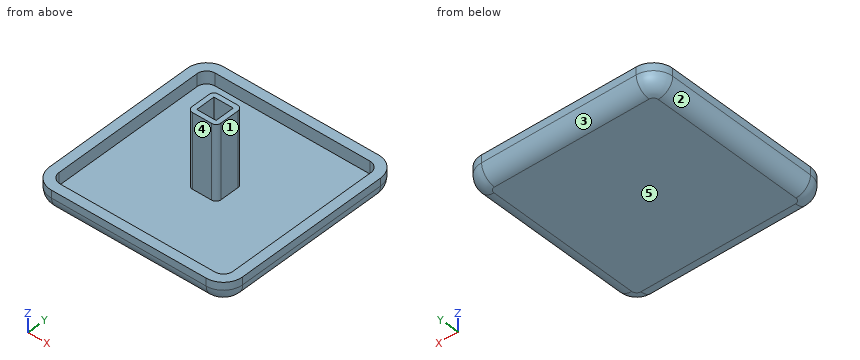
Autodesk Inventor part; units mm, degrees
ref_plane "YZ Plane" through (0, 0, 0) normal (1, 0, 0) x (0, 1, 0)
ref_plane "XZ Plane" through (0, 0, 0) normal (0, 1, 0) x (-1, 0, 0)
ref_plane "XY Plane" through (0, 0, 0) normal (0, 0, 1) x (1, 0, 0)
sketch "Skizze1" plane through (0, 0, 0) normal (0, 0, 1) x (1, 0, 0)
  line L0 (-10, 10) -> (10, 10)
  line L1 (10, 10) -> (10, -10)
  line L2 (10, -10) -> (-10, -10)
  line L3 (-10, -10) -> (-10, 10)
  line L4 (-10, 10) -> (10, -10) construction
  line L5 (10, 10) -> (-10, -10) construction
  point P0 (0, 0)
  dimension "d0" = 20
  dimension "d1" = 20
extrude "Extrusion1" add sketch "Skizze1" along normal blind 2.3
fillet "Rundung1" radius 2 4 edges at (10, 10, 1.15) (-10, 10, 1.15) (10, -10, 1.15) (-10, -10, 1.15)
shell "Wandung1" thickness 1 removed faces 1 at (-2.6667, -2, 2.3)
fillet "Rundung2" radius 1.5 8 edges at (-9.4142, 9.4142, 0) (-10, 0, 0) (-9.4142, -9.4142, 0) (0, -10, 0) (9.4142, -9.4142, 0) (10, 0, 0) (9.4142, 9.4142, 0) (0, 10, 0)
sketch "Skizze2" plane through (-9, 9, 1) normal (0, 0, 1) x (1, 0, 0)
  line L0 (7.5, -7.5) -> (10.5, -7.5)
  line L1 (10.5, -7.5) -> (10.5, -10.5)
  line L2 (10.5, -10.5) -> (7.5, -10.5)
  line L3 (7.5, -10.5) -> (7.5, -7.5)
  line L4 (7.5, -7.5) -> (10.5, -10.5) construction
  line L5 (10.5, -7.5) -> (7.5, -10.5) construction
  point P0 (9, -9)
  dimension "d7" = 3
  dimension "d8" = 3
extrude "Extrusion2" add sketch "Skizze2" along normal blind 7.7
fillet "Rundung3" radius 0.5 4 edges at (1.5, 1.5, 4.85) (-1.5, 1.5, 4.85) (1.5, -1.5, 4.85) (-1.5, -1.5, 4.85)
shell "Wandung2" thickness 0.5 removed faces 1 at (0.3333, -0.5, 8.7)
properties part number "Abdeckkappe 5 20x20"
Here's how the part is built. I have some questions about the finished solid (model axes, mm). Face numbers are marked on the shaded views. A direction names the side the tool comes from. Round coordinates to 2 decimals unless told otherwise and drop trailing zeros. Order: outer loops, then holes, each group sorted by start corner. A loop starts at its lowest first (then second) coordinate and runs counter-clockwise, first axis right, second up. Notation, with made-up numbers: M 9.25,-16 L 63.25,-16 A28 ccw 63.25,20 Z; hole C -8.5,85 d3. An arc over 180 degrees is marked long. Answer in a Markdown table with one row per item.
Item 1: Imagine slicing it at B-B, the plane z = 4.75. Write out the boundary of the cut face in (x, y).
A:
| item | result |
|---|---|
| outline | M -1.5,-1 A0.5 ccw -1,-1.5 L 1,-1.5 A0.5 ccw 1.5,-1 L 1.5,1 A0.5 ccw 1,1.5 L -1,1.5 A0.5 ccw -1.5,1 Z; hole M -1,-1 L 1,-1 L 1,1 L -1,1 Z |
Item 2: Thinking about a two-plate mould opening in X: for the marked faces 1, 2 and 3, which applies, +X half, -X half, draft (parallel to the pull), parting line (faces both ways), or undercut?
A:
| item | result |
|---|---|
| face 1 | undercut |
| face 2 | -X half |
| face 3 | draft |
Item 3: For the marked faces 4 and 5, which set-ups out of +Z, -Z, +X, -X, +Y, -Y let a thin tool reach every point of the face, with its end or its side?
A:
| item | result |
|---|---|
| face 4 | +Z |
| face 5 | -Z, +X, -X, +Y, -Y |
Item 4: Imagine slicing it at C-C, the plane x = 5.25. Write out the boundary of the cut face in (y, z), and give its area (3 significant figures).
A:
| item | result |
|---|---|
| outline | M -10,1.5 A1.5 ccw -8.5,0 L 8.5,0 A1.5 ccw 10,1.5 L 10,2.3 L 9,2.3 L 9,1 L -9,1 L -9,2.3 L -10,2.3 Z |
| area | 21.6 mm2 |
Item 5: Imagine slicing it at A-A, the plane z = 2. Write out the boundary of the cut face in (x, y), and give its area (3 significant figures).
A:
| item | result |
|---|---|
| outline | M -10,-8 A2 ccw -8,-10 L 8,-10 A2 ccw 10,-8 L 10,8 A2 ccw 8,10 L -8,10 A2 ccw -10,8 Z; M -1.5,-1 A0.5 ccw -1,-1.5 L 1,-1.5 A0.5 ccw 1.5,-1 L 1.5,1 A0.5 ccw 1,1.5 L -1,1.5 A0.5 ccw -1.5,1 Z; hole M -9,-8 A1 ccw -8,-9 L 8,-9 A1 ccw 9,-8 L 9,8 A1 ccw 8,9 L -8,9 A1 ccw -9,8 Z; hole M -1,-1 L 1,-1 L 1,1 L -1,1 Z |
| area | 78.2 mm2 |
Item 6: I'm going to push flat-ended pins straight in: pin 1 (0.6 mm diameter, centred on y = 0, z = 5.5, fed in from -X); pin 2 (5 mm diameter, centred on x = -7.5, y = -2, fed in from +Z); pin 3 (1 mm diameter, centred on y = 0.5, z = 5.5, fed in from +X); pin 4 (2 mm diameter, centred on y = -7.5, z = 4.5, fed in from -X). Where does each tip first touch, or does it pass through?
A:
| item | result |
|---|---|
| pin 1 | stops at x = -1.5 |
| pin 2 | stops at z = 2.3 |
| pin 3 | stops at x = 1.5 |
| pin 4 | passes through |
Item 7: If I drill on L1, parallel to Y at x = -0.5, z = 8.5; L2, parallel to Y at x = -8, z = 1.5; L3, parallel to Z at x = -7.5, y = 5.25, over which ranges is the centre line in solid material (lowest first)? Write a range as from..to.
A:
| item | result |
|---|---|
| L1 | y = -1.5..-1, 1..1.5 |
| L2 | y = -10..-9, 9..10 |
| L3 | z = 0..1 |
